from build123d import *

# Parameters (mm, degrees)
F1_DEPTH = 15
F2_W     = 5
F2_H     = 12.9289321881
F3_DEPTH = 25
F4_W     = 12.9289321881
F4_H     = 5
F5_DEPTH = 25
F6_R     = 2.49999
F7_R     = 2.5
F8_DEPTH = 25


# Not quite as in the source:
# - a fillet or chamfer is up to 0.001 mm smaller than in the source, because OpenCascade refuses the exact size


with BuildPart() as f1:
    # F0 (on Front) → F1 (new body)
    with BuildSketch(Plane.XZ):
        with BuildLine():
            Line((2.5, 25), (-2.5, 25))
            Line((-2.5, 25), (-2.5, 7.0710678119))
            ThreePointArc((-2.5, 7.0710678119), (-5.3033008589, -5.3033008589), (7.0710678119, -2.5))
            Line((7.0710678119, -2.5), (25, -2.5))
            Line((25, -2.5), (25, 2.5))
            Line((25, 2.5), (7.0710678119, 2.5))
            ThreePointArc((7.0710678119, 2.5), (5.3033008589, 5.3033008589), (2.5, 7.0710678119))
            Line((2.5, 7.0710678119), (2.5, 25))
        make_face()
    extrude(amount=F1_DEPTH)

    # F2 (on face) → F3 (cut)
    with BuildSketch(Plane.YZ.offset(2.5)):
        with Locations((-7.5, 13.5355339059)):
            Rectangle(F2_W, F2_H)
    extrude(amount=-F3_DEPTH, mode=Mode.SUBTRACT)

    # F4 (on face) → F5 (cut)
    with BuildSketch(Plane.XY.offset(2.5)):
        with Locations((13.5355339059, -7.5)):
            Rectangle(F4_W, F4_H)
    extrude(amount=-F5_DEPTH, mode=Mode.SUBTRACT)

    # F6 (radius 2.5 in the source; OpenCascade refuses exactly that, so slightly less here)
    f6_edges = [f1.edges().sort_by_distance(p)[0] for p in [
        (-2.5, -7.5, 25),
        (2.5, -7.5, 25),
        (-2.5, -7.5, 20),
        (2.5, -7.5, 20),
        (25, -7.5, -2.5),
        (25, -7.5, 2.5),
        (20, -7.5, -2.5),
        (20, -7.5, 2.5),
    ]]
    fillet(f6_edges, radius=F6_R)

    # F7 (on face) → F8 (cut)
    with BuildSketch(Plane.XZ.offset(15)):
        Circle(F7_R)
    extrude(amount=-F8_DEPTH, mode=Mode.SUBTRACT)


solid = f1.part
Input: part model. Units: mm. Frame: model coordinates. A direction names the side the tool comes from. Coordinates: 2 decimals unless noted, no trailing zeros. Order: outer loops, then holes, each group sorted by start corner. A loop starts at its lowest first (then second) coordinate and runs counter-clockwise, first axis right, second up. Notation, with made-up numbers: M 22.5,12 L 62.5,12 A9 cw 62.5,25 Z; hole C -23.5,7 d1. An arc over 180 degrees is marked long. Write item = value, one per line. Start each with the question number.
(1) First-contact query: P1, Ø1.5, axis at y = -8, z = -1, coming from the +X side; P2, Ø3, axis at y = -6, z = 3, coming from the +X side; P3, Ø4.5, axis at x = 0, z = 0, coming from the +Y side; P4, Ø7.5, axis at x = 15, y = -4, coming from the -Z side. Flat tips, straight axial feed; report the tip coordinate or a pass-through.
(2) Section A-A on y = -9.5. Give the number of separate pieces and of enclosed holes in the cut face, and give its area (3 significant figures).
(3) Section C-C on z = 2. Output: boundary loops of the cut face in (x, y), and give its area (3 significant figures).
(4) Section B-B on x = 18. Output: boundary loops of the cut face in (y, z), and give its area (3 significant figures).
(5) Line query: line 1 along Z through (x, y) = (0, -9); line 2 along Z through (x, y) = (0, -11.75); line 3 along Z through (x, y) = (13.5, -10.5). Output: solid intervals per line, ascending. Write a range as [from, to].
(6) Pull-direction query (Y, two-part tool) for faces 1 (the flat face through (5, -15, 5)), 2 (the flat face through (15, -4, 2.5)), 3 (the flat face through (5, 0, 5)), 4 (the flat face through (0, -10, 13)); classes: released by +Y, released by -Y, zero draft, split by the parting line, or undercut.
(7) Reachability of faces 5 (the cylindrical face through (21, -7, 2)), 6 (the flat face through (0, -8, 7.071)), 7 (the flat face through (15, -4, -2.5)), 8 (the cylindrical face through (-2, -7, 21)) from +Z, -Z, +X, -X, +Y, -Y: full face, straight path, thin tool, end or side. Return the list, or none.
Result set:
q1.P1 = 24.99
q1.P2 = 24.5
q1.P3 = through
q1.P4 = -2.5
q2.separate_pieces = 3
q2.enclosed_holes = 1
q2.area = 193 mm²
q3.outline = M -7.23,-15 L -1.5,-15 L -1.5,0 L -7.23,0 Z; M 1.5,-15 L 24,-15 L 24,0 L 1.5,0 Z; hole M 7.07,-10 L 21,-10 L 21,-5 L 7.07,-5 Z
q3.area = 354 mm²
q4.outline = M -15,-2.5 L -10,-2.5 L -10,2.5 L -15,2.5 Z; M -5,-2.5 L 0,-2.5 L 0,2.5 L -5,2.5 Z
q4.area = 50.0 mm²
q5.line_1 = [-7.5, -2.5], [2.5, 7.07], [20, 25]
q5.line_2 = [-7.5, -2.5], [2.5, 25]
q5.line_3 = [-2.5, 2.5]
q6.face_1 = released by -Y
q6.face_2 = zero draft
q6.face_3 = released by +Y
q6.face_4 = undercut
q7.face_5 = +Z
q7.face_6 = +X, -X
q7.face_7 = -Z, +X, +Y, -Y
q7.face_8 = -X
